```python
from build123d import *

# Parameters (mm, degrees)
EXTRUDE1_DEPTH  = 76.2
FILLET1_R       = 1.190625
SKETCH4_R       = 2.1463
EXTRUDE3_DEPTH  = 4.7625
LPATTERN1_COUNT = 19
LPATTERN1_PITCH = 101.6


with BuildPart() as part:
    # Sketch1 → Extrude1 (new body, symmetric)
    with BuildSketch(Plane.XY):
        with BuildLine():
            Line((-19.05, 0), (19.05, 0))
            Line((19.05, 0), (19.05, 4.7625))
            Line((19.05, 4.7625), (5.585983612, 4.7625))
            Line((5.585983612, 4.7625), (3.175, 13.760413336))
            Line((3.175, 13.760413336), (3.175, 23.075738686))
            ThreePointArc((3.175, 23.075738686), (0, 34.925), (-3.175, 23.075738686))
            Line((-3.175, 23.075738686), (-3.175, 13.760413336))
            Line((-3.175, 13.760413336), (-5.585983612, 4.7625))
            Line((-5.585983612, 4.7625), (-19.05, 4.7625))
            Line((-19.05, 4.7625), (-19.05, 0))
        make_face()
    extrude(amount=EXTRUDE1_DEPTH, both=True)

    # Sketch3 → Cut-Revolve1 (revolve, cut)
    with BuildSketch(Plane(origin=(0, 0, 0), x_dir=(0, 0, -1), z_dir=(1, 0, 0))):
        Polygon((-76.2, 33.9725), (-75.2475, 34.925), (-76.2, 34.925), align=None)
    cut_revolve1 = revolve(axis=Axis((0, 28.575, 76.2), (0, 0, -1)), mode=Mode.SUBTRACT)

    # Mirror1: Cut-Revolve1 across plane
    add(cut_revolve1.mirror(Plane.XY), mode=Mode.SUBTRACT)

    # Fillet1
    fillet1_edges = [part.edges().sort_by_distance(p)[0] for p in [
        (-19.05, 4.7625, 0),
        (19.05, 4.7625, 0),
    ]]
    fillet(fillet1_edges, radius=FILLET1_R)

    # Sketch4 → Extrude3 (cut)
    with BuildSketch(Plane(origin=(0, 0, 0), x_dir=(1, 0, 0), z_dir=(0, 1, 0))):
        with Locations((12.7, -50.8)):
            Circle(SKETCH4_R)
        with Locations((-12.7, -50.8)):
            Circle(SKETCH4_R)
    extrude3 = extrude(amount=EXTRUDE3_DEPTH, mode=Mode.SUBTRACT)

    # LPattern1: Extrude3 ×19
    with Locations(*[(0, 0, -i * LPATTERN1_PITCH) for i in range(1, LPATTERN1_COUNT)]):
        add(extrude3, mode=Mode.SUBTRACT)


solid = part.part
```
Could you check a few things on this model? Use its own coordinates, in mm. A direction names the side the tool comes from. Round coordinates to 2 decimals unless told otherwise and drop trailing zeros. Write each loop counter-clockwise with the first axis right and the second up, starting at its lowest first coordinate (ties: lowest second). Pieces come first, ordered by that corner, then holes.
(1) Suppose I cut it at B-B on x = -12.7. Write out the boundary of the cut face in (y, z).
Findings below:
outline: (0, -76.2) - (4.76, -76.2) - (4.76, -52.95) - (0, -52.95) - close; (0, -48.65) - (4.76, -48.65) - (4.76, 48.65) - (0, 48.65) - close; (0, 52.95) - (4.76, 52.95) - (4.76, 76.2) - (0, 76.2) - close
(2) If I drill on probe 1 along Z at (x, y) = (-12.7, 2.7); probe 2 along X at (y, z) = (1.35, -50.8); probe 3 along Z at (x, y) = (-12, 3), over which ranges is the centre line in solid material (lowest first)?
Findings below:
probe 1: z = -76.2 to -52.95, -48.65 to 48.65, 52.95 to 76.2
probe 2: x = -19.05 to -14.85, -10.55 to 10.55, 14.85 to 19.05
probe 3: z = -76.2 to -52.83, -48.77 to 48.77, 52.83 to 76.2
(3) Suppose I cut it at A-A on z = 50.8. State how many separate pieces and enclosed holes the cut face has, and give its area (3 significant figures).
Findings below:
separate pieces: 3
enclosed holes: 0
area: 401 mm2
(4) Which directions (+Z, -Z, +X, -X, +Y, -Y) give clear straight access to the entire face, cutting with the end or side of a thin tool? Please do faces 4 (the face through (-12, 4.762, 1)), 5 (the face through (-19.05, 2, 1)), 6 (the face through (3.175, 18, 1)).
Findings below:
face 4: +Z, -Z, -X
face 5: +Z, -Z, -X, +Y, -Y
face 6: +Z, -Z, +X
(5) Thinking about a two-plate mould opening in Y: for faces 1 (the face through (0, 0, 1)), 2 (the face through (4.397, 9.198, 1.067)), 3 (the face through (-11.7, 2.3, 52.7)), which applies, +Y half, -Y half, draft (parallel to the pull), parting line (faces both ways), or undercut?
Findings below:
face 1: -Y half
face 2: undercut
face 3: draft
(6) For pin 1 (8 mm diameter, centred on y = 26, z = 6.5, fed in from +X); pin 2 (7.5 mm diameter, centred on y = 18.5, z = -32.5, fed in from +X) (3 decimals); pin 3 (10 mm diameter, centred on x = 9.5, z = 3.5, fed in from +Y), each with a flat end and sliding along its axis, tell me the tip position at first contact or that it passes through.
Findings below:
pin 1: stops at x = 6.35
pin 2: stops at x = 3.175
pin 3: stops at y = 33.06
(7) Suppose I cut it at D-D on y = 16.5. Write out the boundary of the cut face in (x, z) (3 decimals).
Findings below:
outline: (-3.175, -76.2) - (3.175, -76.2) - (3.175, 76.2) - (-3.175, 76.2) - close
